from build123d import *

# Parameters (mm, degrees)
BOSS_EXTRUDE1_DEPTH = 3.6
SKETCH3_R           = 2.5
BOSS_EXTRUDE2_DEPTH = 31.5
CHAMFER1_SIZE       = 0.5
FILLET1_R           = 0.4


with BuildPart() as part:
    # Sketch1 → Boss-Extrude1 (new body)
    with BuildSketch(Plane(origin=(0, 0, 0), x_dir=(1, 0, 0), z_dir=(0, 1, 0))):
        Polygon((-2.309401077, -4), (2.309401077, -4), (4.618802154, 0), (2.309401077, 4), (-2.309401077, 4), (-4.618802154, 0), align=None)
    extrude(amount=BOSS_EXTRUDE1_DEPTH)

    # Sketch2 → Cut-Revolve1 (revolve, cut)
    with BuildSketch(Plane(origin=(0, 0, 0), x_dir=(0, 0, -1), z_dir=(1, 0, 0))):
        Polygon((8.326224825, 1.102252933), (4, 3.6), (8.326224825, 3.6), align=None)
    revolve(axis=Axis((0, 0, 0), (0, 1, 0)), mode=Mode.SUBTRACT)

    # Sketch3 → Boss-Extrude2 (add)
    with BuildSketch(Plane.XZ):
        Circle(SKETCH3_R)
    extrude(amount=BOSS_EXTRUDE2_DEPTH)

    # Chamfer1
    chamfer1_edges = [part.edges().sort_by_distance(p)[0] for p in [
        (-2.5, -31.5, 0),
    ]]
    chamfer(chamfer1_edges, length=CHAMFER1_SIZE)

    # Fillet1
    fillet1_edges = [part.edges().sort_by_distance(p)[0] for p in [
        (-2.5, 0, 0),
    ]]
    fillet(fillet1_edges, radius=FILLET1_R)


solid = part.part
The listing builds one solid part. Answer for the finished solid, in the listing's coordinates (mm). A direction names the side the tool comes from. Give positions to 0.01 mm unless a question says otherwise; leave off trailing zeros. Order: outer loops, then holes, each group sorted by start corner. A loop starts at its lowest first (then second) coordinate and runs counter-clockwise, first axis right, second up. Notation, with made-up numbers: (46, 45) - (73, 45) arc R14 cw to (73, 71) - close; hole circle Ø8 at (74, 73.25). An arc over 180 degrees is marked (long way). Use one line per item in the form item = value.
1) Consider probe 1 along Y at (x, z) = (2.5, -2); probe 2 along Z at (x, y) = (-1.5, -3.5); probe 3 along X at (y, z) = (-25, -2). Determine where each line is inside the solid, lowest interval first. Write a range as [from, to].
Verdict:
probe_1 = [0, 3.6]
probe_2 = [-2, 2]
probe_3 = [-1.5, 1.5]
2) Find section A-A on y = -21. Determine the outline of the cut face in (x, z).
Verdict:
outline = circle Ø5 at (0, 0)
3) For faces 1 (the cylindrical face through (-0.54, -15.49, -2.44)), 2 (the flat face through (3.448, 1.775, 2.028)), determine the directions among +Z, -Z, +X, -X, +Y, -Y from which every point of the face is accessible in a straight line to the end or side of a thin tool.
Verdict:
face_1 = -Y
face_2 = +Z, +X, +Y, -Y
4) Each of these flat-tipped pins is pushed along its axis until it touches: pin 1 (1.5 mm diameter, centred on y = -23.5, z = 1, fed in from +X); pin 2 (5 mm diameter, centred on x = -2.5, y = -20, fed in from +Z); pin 3 (1 mm diameter, centred on x = -3.5, y = -5.5, fed in from -Z) (3 decimals). Where does it stop, or does it pass through?
Verdict:
pin_1 = 2.49
pin_2 = 2.5
pin_3 = through
